from build123d import *

# Parameters (mm, degrees)
EXTRUDE_1_DEPTH          = 170
SKETCH_2_R               = 60
CUT_EXTRUDE_1_DEPTH      = 180
CUT_EXTRUDE_2_DEPTH      = 313.955268369
CUT_EXTRUDE_2_DEPTH_BACK = 313.955268369
SKETCH_3_R               = 11
FILLET_1_R               = 70
FILLET_2_R               = 5
FILLET_3_R               = 10
SKETCH_6_R               = 30
CUT_EXTRUDE_6_DEPTH      = 39
SKETCH_7_R               = 13
CUT_EXTRUDE_7_DEPTH      = 0.7


with BuildPart() as part:
    # 草图1 → 凸台-拉伸1 (new body)
    with BuildSketch(Plane.XY):
        Polygon((-180, 0), (0, 0), (0, -175), (8, -175), (8, 8), (-180, 8), (-188, 8), (-188, -175), (-180, -175), align=None)
    extrude(amount=EXTRUDE_1_DEPTH)

    # 草图2 → 切除-拉伸1 (cut)
    with BuildSketch(Plane(origin=(0, 8, 0), x_dir=(1, 0, 0), z_dir=(0, 1, 0))):
        with Locations(Location((-90, -85, 0), (0, 0, 180))):
            Circle(SKETCH_2_R)
    extrude(amount=-CUT_EXTRUDE_1_DEPTH, mode=Mode.SUBTRACT)

    # 草图3 → 切除-拉伸2 (cut, two sides: drawn at the far end of the back side and taken through both)
    with BuildSketch(Plane(origin=(8, 0, 0), x_dir=(0, 0, -1), z_dir=(1, 0, 0)).offset(-CUT_EXTRUDE_2_DEPTH_BACK)):
        with Locations(Location((-85, -95, 0), (0, 0, 90))):
            Circle(SKETCH_3_R)
    extrude(amount=CUT_EXTRUDE_2_DEPTH + CUT_EXTRUDE_2_DEPTH_BACK, mode=Mode.SUBTRACT)

    # 圆角1
    fillet_1_edges = [part.edges().sort_by_distance(p)[0] for p in [
        (4, -175, 0),
        (4, -175, 170),
        (-184, -175, 170),
        (-184, -175, 0),
    ]]
    fillet(fillet_1_edges, radius=FILLET_1_R)

    # 圆角2
    fillet_2_edges = [part.edges().sort_by_distance(p)[0] for p in [
        (0, 0, 85),
        (-180, 0, 85),
    ]]
    fillet(fillet_2_edges, radius=FILLET_2_R)

    # 圆角3
    fillet_3_edges = [part.edges().sort_by_distance(p)[0] for p in [
        (-188, 8, 85),
        (8, 8, 85),
    ]]
    fillet(fillet_3_edges, radius=FILLET_3_R)

    # 草图6 → 切除-拉伸6 (cut)
    with BuildSketch(Plane.ZY.offset(188)):
        with Locations(Location((85, -95, 0), (0, 0, 270))):
            Circle(SKETCH_6_R)
    extrude(amount=-CUT_EXTRUDE_6_DEPTH, mode=Mode.SUBTRACT)

    # 草图7 → 切除-拉伸7 (cut)
    with BuildSketch(Plane.ZY):
        with Locations(Location((85, -95, 0), (0, 0, 270))):
            Circle(SKETCH_7_R)
    extrude(amount=-CUT_EXTRUDE_7_DEPTH, mode=Mode.SUBTRACT)


solid = part.part
Design review of the part built by this model. Coordinates are the model's own, in mm. A direction names the side the tool comes from. Coordinates: 2 decimals unless noted, no trailing zeros. Loops run counter-clockwise (first coordinate to the right, second up) from the corner with the lowest first, then second, coordinate; pieces in that order, holes last. Notation, with made-up numbers: M -3,89 L 29,89 A23 ccw 29,124 Z; hole C -26.5,74 d2. An arc over 180 degrees is marked long. Answer as CSV lines item,"result".
Item 1: For probe 1 along X at (y, z) = (-23.5, 153.5); probe 2 along Z at (x, y) = (-182, -95); probe 3 along X at (y, z) = (-75, 83), list the stretches that pass through material, from the lowest coordinate up.
Answer list:
probe 1,"-188 to -180, 0 to 8"
probe 2,"0 to 55, 115 to 170"
probe 3,"0 to 8"
Item 2: Add section C-C on y = -161. State the section outline as (x, z) points, plus the area to 3 significant figures.
Answer list:
outline,"M -188,28 L -180,28 L -180,142 L -188,142 Z; M 0,28 L 8,28 L 8,142 L 0,142 Z"
area,"1,820 mm²"
Item 3: For P1, Ø21, axis at y = -95, z = 85, coming from the -X side; P2, Ø8, axis at y = -80, z = 66, coming from the -X side, all flat-tipped, find the tip position at first contact; note any pin that passes through.
Answer list:
P1,"through"
P2,"x = 0"
Item 4: The part is to be moulded in two halves that separate along Z. For faces 1 (the face through (4.06, -153.95, 150.04)), 2 (the face through (4, -106, 85)), 3 (the face through (-179, -2, 86)), say which applies: pulls with the +Z half, pulls with the -Z half, needs draft (parallel to the pull), parting line crosses it, or undercut.
Answer list:
face 1,"pulls with the +Z half"
face 2,"undercut"
face 3,"needs draft"
Item 5: Add section A-A on x = -90. State the section outline as (y, z) points.
Answer list:
outline,"M 0,0 L 8,0 L 8,25 L 0,25 Z; M 0,145 L 8,145 L 8,170 L 0,170 Z"
Item 6: Add section B-B on z = 85. State the section outline as (x, y) points.
Answer list:
outline,"M -188,-175 L -180,-175 L -180,-125 L -188,-125 Z; M -188,-65 L -180,-65 L -180,-5 A5 cw -175,0 L -150,0 L -150,8 L -178,8 A10 ccw -188,-2 Z; M -30,0 L -5,0 A5 cw 0,-5 L 0,-82 L 0.7,-82 L 0.7,-84 L 8,-84 L 8,-2 A10 ccw -2,8 L -30,8 Z; M 0,-175 L 8,-175 L 8,-106 L 0.7,-106 L 0.7,-108 L 0,-108 Z"
Item 7: Machinability: for faces 4 (the face through (-180, -72, 65)), 5 (the face through (-98, 2, 170)), 6 (the face through (0.7, -84, 88)), which of the approach directions +Z, -Z, +X, -X, +Y, -Y give a long, thin tool a straight path to every point of the face, cutting with its end or side? Answer none if there is none.
Answer list:
face 4,"+Z, -Z, -Y"
face 5,"+Z, +X, -X, +Y, -Y"
face 6,"-X"
Item 8: Add section D-D on y = -95. State the section outline as (x, z) points.
Answer list:
outline,"M -188,0 L -180,0 L -180,55 L -188,55 Z; M -188,115 L -180,115 L -180,170 L -188,170 Z; M 0,0 L 8,0 L 8,74 L 0.7,74 L 0.7,72 L 0,72 Z; M 0,98 L 0.7,98 L 0.7,96 L 8,96 L 8,170 L 0,170 Z"
